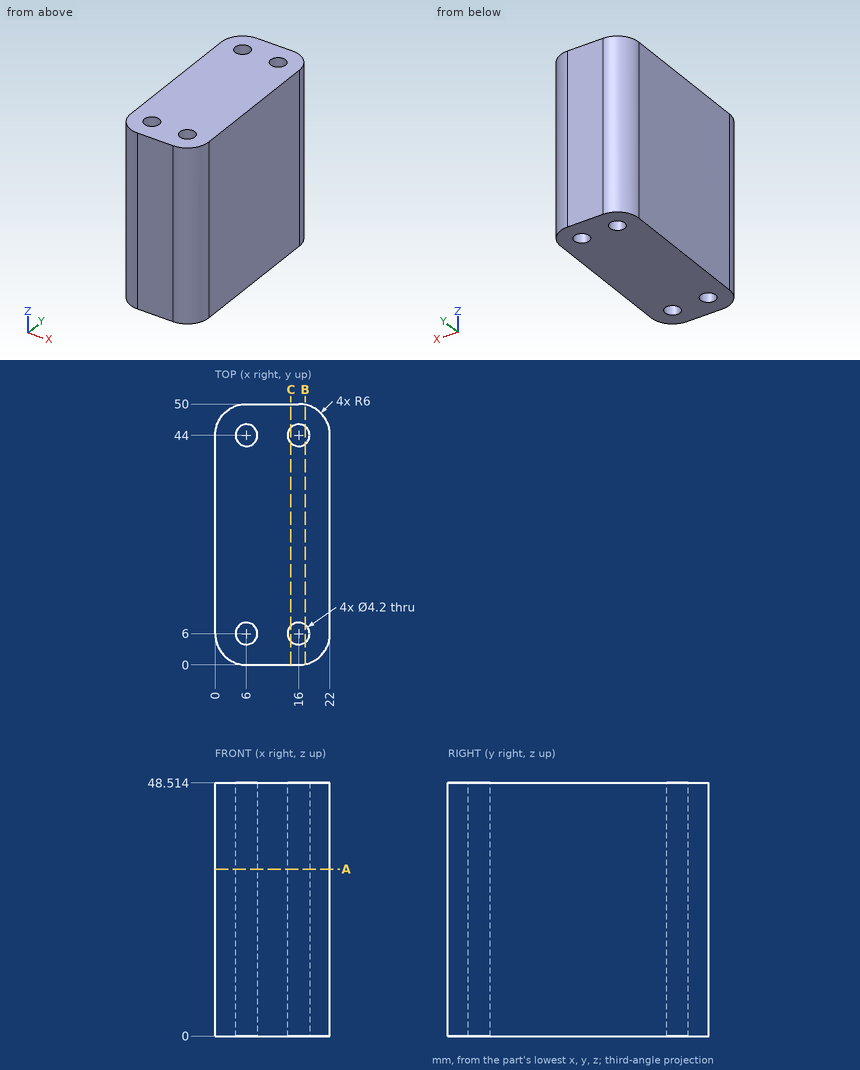
Geometry: see drawing. Coordinates: mm, zero at the bounding-box minimum. Coordinates: 2 decimals unless noted, no trailing zeros. Loops run counter-clockwise (first coordinate to the right, second up) from the corner with the lowest first, then second, coordinate; pieces in that order, holes last. Notation, with made-up numbers: M 44.25,22.5 L 86.25,22.5 A29 cw 86.25,57.5 Z; hole C -29.5,39 d8. An arc over 180 degrees is marked long. Answer in a Markdown table with one row per item.
1. Section C-C, the plane x = 14.5. Output: boundary loops of the cut face in (y, z).
Response:
| item | result |
|---|---|
| outline | M 0,0 L 4.53,0 L 4.53,48.51 L 0,48.51 Z; M 7.47,0 L 42.53,0 L 42.53,48.51 L 7.47,48.51 Z; M 45.47,0 L 50,0 L 50,48.51 L 45.47,48.51 Z |
2. First-contact query: pin 1 (4 mm diameter, centred on y = 34.5, z = 21, fed in from -X); pin 2 (2.5 mm diameter, centred on x = 6, y = 6, fed in from +Z). Flat tips, straight axial feed; report the tip coordinate or a pass-through.
Response:
| item | result |
|---|---|
| pin 1 | stops at x = 0 |
| pin 2 | passes through |
3. Section A-A, the plane z = 32. Output: boundary loops of the cut face in (x, y), then the cut area to 3 significant figures.
Response:
| item | result |
|---|---|
| outline | M 0,6 A6 ccw 6,0 L 16,0 A6 ccw 22,6 L 22,44 A6 ccw 16,50 L 6,50 A6 ccw 0,44 Z; hole C 6,6 d4.2; hole C 6,44 d4.2; hole C 16,6 d4.2; hole C 16,44 d4.2 |
| area | 1,010 mm2 |
4. Section B-B, the plane x = 17.25. Output: boundary loops of the cut face in (y, z), then the cut area to 3 significant figures.
Response:
| item | result |
|---|---|
| outline | M 0.13,0 L 4.31,0 L 4.31,48.51 L 0.13,48.51 Z; M 7.69,0 L 42.31,0 L 42.31,48.51 L 7.69,48.51 Z; M 45.69,0 L 49.87,0 L 49.87,48.51 L 45.69,48.51 Z |
| area | 2,090 mm2 |
5. Material intervals for line 1 (Y direction, x = 16, z = 18.5); line 2 (Y direction, x = 7.5, z = 13); line 3 (X direction, y = 7, z = 35), sorted ascending.
Response:
| item | result |
|---|---|
| line 1 | y = 0 to 3.9, 8.1 to 41.9, 46.1 to 50 |
| line 2 | y = 0 to 4.53, 7.47 to 42.53, 45.47 to 50 |
| line 3 | x = 0 to 4.15, 7.85 to 14.15, 17.85 to 22 |
